The listing builds one solid part. Answer for the finished solid, in the listing's coordinates (mm). A direction names the side the tool comes from. Coordinates: 2 decimals unless noted, no trailing zeros. Write each loop counter-clockwise with the first axis right and the second up, starting at its lowest first coordinate (ties: lowest second). Pieces come first, ordered by that corner, then holes.
from build123d import *

# Parameters (mm, degrees)
F1_DEPTH = 25.4
F4_DEPTH = 25.4
F6_DEPTH = 25.4
F7_R     = 10.7031711433
F7_R_2   = 10.853136357
F8_DEPTH = 25.4


with BuildPart() as f1:
    # F0 (on Front) → F1 (new body)
    with BuildSketch(Plane.XZ):
        Polygon((-20.5684766621, 44.45), (-33.2684766621, 44.45), (-33.2684766621, 0), (42.9315233379, 0), (42.9315233379, 12.7), (-20.5684766621, 12.7), align=None)
    extrude(amount=F1_DEPTH)

    # F3 (on face) → F4 (cut)
    with BuildSketch(Plane.YZ.offset(-20.5684766621)):
        with BuildLine():
            ThreePointArc((-25.4, 29.5939260799), (-12.5203138917, 40.7445202451), (0, 29.1918666739))
            Line((0, 29.1918666739), (0, 44.45))
            Line((0, 44.45), (-25.4, 44.45))
            Line((-25.4, 44.45), (-25.4, 29.5939260799))
        make_face()
    extrude(amount=-F4_DEPTH, mode=Mode.SUBTRACT)

    # F5 (on face) → F6 (cut)
    with BuildSketch(Plane.YZ.offset(-20.5684766621)):
        with BuildLine():
            ThreePointArc((-6.1516358245, 38.9277270751), (-12.5777297237, 40.7453000896), (-19.0433743714, 39.0738654502))
            ThreePointArc((-19.0433743714, 39.0738654502), (-12.7443611857, 26.0457440008), (-6.1516358245, 38.9277270751))
        make_face()
    extrude(amount=-F6_DEPTH, mode=Mode.SUBTRACT)

    # F7 (on face) → F8 (cut)
    with BuildSketch(Plane.XY.offset(12.7)):
        with Locations((-6.5744994208, -11.0673578456)):
            Circle(F7_R)
        with Locations((15.5932949856, -11.4149535075)):
            Circle(F7_R_2)
    extrude(amount=-F8_DEPTH, mode=Mode.SUBTRACT)


solid = f1.part
1. Section D-D on x = -27 is taken. Give the vertices of the cut face in (y, z), then the cut area to 3 significant figures.
Results found:
outline: (-25.4, 0) - (0, 0) - (0, 29.19) arc R12.78 ccw to (-6.15, 38.93) arc R8.08 cw (long way) to (-19.04, 39.07) arc R12.78 ccw to (-25.4, 29.59) - close
area: 775 mm2
2. Section B-B on z = 33.5 is taken. Give the vertices of the cut face in (x, y), then the cut area to 3 significant figures.
Results found:
outline: (-33.27, -24.24) - (-20.57, -24.24) - (-20.57, -20.71) - (-33.27, -20.71) - close; (-33.27, -4.6) - (-20.57, -4.6) - (-20.57, -1.2) - (-33.27, -1.2) - close
area: 88.0 mm2
3. Section A-A on x = -16.5 is taken. Give the vertices of the cut face in (y, z).
Results found:
outline: (-25.4, 0) - (-15.07, 0) - (-15.07, 12.7) - (-25.4, 12.7) - close; (-7.06, 0) - (0, 0) - (0, 12.7) - (-7.06, 12.7) - close
4. For a pull along Z with two mould halves and no side action, classify faces 1 (the flat face through (26, -15, 12.7)), 2 (the flat face through (4.3, -12.5, 0)), 3 (the flat face through (-4, -25.4, 8)), 4 (the cylindrical face through (-26.83, -12.995, 26.052)) as pulls with the +Z half, pulls with the -Z half, needs draft (parallel to the pull), parting line crosses it, or undercut.
Results found:
face 1: pulls with the +Z half
face 2: pulls with the -Z half
face 3: needs draft
face 4: undercut
5. Find the intervals of material crossed by L1, parallel to X at y = -14, z = 9; L2, parallel to X at y = -10.5, z = 10; L3, parallel to Z at x = 38.5, y = -3.25, in increasing order.
Results found:
L1: x = -33.27 to -16.87, 3.72 to 5.05, 26.13 to 42.93
L2: x = -33.27 to -17.26, 4.11 to 4.78, 26.41 to 42.93
L3: z = 0 to 12.7
6. A tool of negligible diameter and unlimited length cuts with its end or side. For faces 5 (the flat face through (-20.568, -13, 23)), 6 (the flat face through (42.932, -13, 6)), from which of +Z, -Z, +X, -X, +Y, -Y can it reach the whole face along a straight path? Write none if from no direction.
Results found:
face 5: +Z, +X, +Y, -Y
face 6: +Z, -Z, +X, +Y, -Y
7. Section C-C on y = -17.25 is taken. Give the vertices of the cut face in (x, z).
Results found:
outline: (-33.27, 0) - (-15.31, 0) - (-15.31, 12.7) - (-20.57, 12.7) - (-20.57, 27.48) - (-33.27, 27.48) - close; (2.16, 0) - (6.44, 0) - (6.44, 12.7) - (2.16, 12.7) - close; (24.74, 0) - (42.93, 0) - (42.93, 12.7) - (24.74, 12.7) - close
8. Flat-ended cylindrical pins translate along their axes: P1, Ø4, axis at y = -21.5, z = 30, coming from the +X side; P2, Ø12.5, axis at x = 3, y = -13.5, coming from the +Z side. Find the tip coordinate at first contact, or state that the pin passes through.
Results found:
P1: stops at x = -20.57
P2: stops at z = 12.7
